Part model, mm, in its own coordinate system. A direction names the side the tool comes from. Give positions to 0.01 mm unless a question says otherwise; leave off trailing zeros. Order: outer loops, then holes, each group sorted by start corner. A loop starts at its lowest first (then second) coordinate and runs counter-clockwise, first axis right, second up. Notation, with made-up numbers: M 25,-24.5 L 53,-24.5 A31 ccw 53,10.5 Z; hole C -3,-2 d2. An arc over 180 degrees is marked long. Answer as a JSON object with one key per item and string values.
from build123d import *

# Parameters (mm, degrees)
SKIZZE1_R                       = 19
SKIZZE1_R_2                     = 1.6
AUFSATZ_LINEAR_AUSTRAGEN1_DEPTH = 3
SKIZZE6_R                       = 3
SCHNITT_LINEAR_AUSTRAGEN2_DEPTH = 36.482389998
SKIZZE7_W                       = 3
SKIZZE7_H                       = 12
SKIZZE7_W_2                     = 12
SKIZZE7_H_2                     = 3
SCHNITT_LINEAR_AUSTRAGEN3_DEPTH = 1.2


with BuildPart() as part:
    # Skizze1 → Aufsatz-Linear austragen1 (new body)
    with BuildSketch(Plane(origin=(0, 0, 0), x_dir=(1, 0, 0), z_dir=(0, 1, 0))):
        with BuildLine():
            ThreePointArc((6, -20.493901532), (6.348554352, -19.365749382), (7.272727273, -18.630819574))
            ThreePointArc((7.272727273, -18.630819574), (14.142135624, -14.142135624), (18.630819574, -7.272727273))
            ThreePointArc((18.630819574, -7.272727273), (19.365749382, -6.348554352), (20.493901532, -6))
            Line((20.493901532, -6), (22.649503306, -6))
            ThreePointArc((22.649503306, -6), (23.93487248, -5.532261755), (24.619025332, -4.347826087))
            ThreePointArc((24.619025332, -4.347826087), (25, 0), (24.619025332, 4.347826087))
            ThreePointArc((24.619025332, 4.347826087), (23.93487248, 5.532261755), (22.649503306, 6))
            Line((22.649503306, 6), (20.493901532, 6))
            ThreePointArc((20.493901532, 6), (19.365749382, 6.348554352), (18.630819574, 7.272727273))
            ThreePointArc((18.630819574, 7.272727273), (14.142135624, 14.142135624), (7.272727273, 18.630819574))
            ThreePointArc((7.272727273, 18.630819574), (6.348554352, 19.365749382), (6, 20.493901532))
            Line((6, 20.493901532), (6, 22.649503306))
            ThreePointArc((6, 22.649503306), (5.532261755, 23.93487248), (4.347826087, 24.619025332))
            ThreePointArc((4.347826087, 24.619025332), (0, 25), (-4.347826087, 24.619025332))
            ThreePointArc((-4.347826087, 24.619025332), (-5.532261755, 23.93487248), (-6, 22.649503306))
            Line((-6, 22.649503306), (-6, 20.493901532))
            ThreePointArc((-6, 20.493901532), (-6.348554352, 19.365749382), (-7.272727273, 18.630819574))
            ThreePointArc((-7.272727273, 18.630819574), (-14.142135624, 14.142135624), (-18.630819574, 7.272727273))
            ThreePointArc((-18.630819574, 7.272727273), (-19.365749382, 6.348554352), (-20.493901532, 6))
            Line((-20.493901532, 6), (-22.649503306, 6))
            ThreePointArc((-22.649503306, 6), (-23.93487248, 5.532261755), (-24.619025332, 4.347826087))
            ThreePointArc((-24.619025332, 4.347826087), (-25, 0), (-24.619025332, -4.347826087))
            ThreePointArc((-24.619025332, -4.347826087), (-23.93487248, -5.532261755), (-22.649503306, -6))
            Line((-22.649503306, -6), (-20.493901532, -6))
            ThreePointArc((-20.493901532, -6), (-19.365749382, -6.348554352), (-18.630819574, -7.272727273))
            ThreePointArc((-18.630819574, -7.272727273), (-14.142135624, -14.142135624), (-7.272727273, -18.630819574))
            ThreePointArc((-7.272727273, -18.630819574), (-6.348554352, -19.365749382), (-6, -20.493901532))
            Line((-6, -20.493901532), (-6, -22.649503306))
            ThreePointArc((-6, -22.649503306), (-5.532261755, -23.93487248), (-4.347826087, -24.619025332))
            ThreePointArc((-4.347826087, -24.619025332), (0, -25), (4.347826087, -24.619025332))
            ThreePointArc((4.347826087, -24.619025332), (5.532261755, -23.93487248), (6, -22.649503306))
            Line((6, -22.649503306), (6, -20.493901532))
        make_face()
        Circle(SKIZZE1_R, mode=Mode.SUBTRACT)
        Circle(SKIZZE1_R)
        with Locations(Location((0, -10, 0), (0, 0, 270))):
            Circle(SKIZZE1_R_2, mode=Mode.SUBTRACT)
        with Locations(Location((-10, 0, 0), (0, 0, 270))):
            Circle(SKIZZE1_R_2, mode=Mode.SUBTRACT)
        with Locations(Location((10, 0, 0), (0, 0, 270))):
            Circle(SKIZZE1_R_2, mode=Mode.SUBTRACT)
        with Locations(Location((0, 10, 0), (0, 0, 270))):
            Circle(SKIZZE1_R_2, mode=Mode.SUBTRACT)
        with Locations(Location((0, 0, 0), (0, 0, 270))):
            Circle(SKIZZE1_R_2, mode=Mode.SUBTRACT)
    extrude(amount=AUFSATZ_LINEAR_AUSTRAGEN1_DEPTH)

    # Skizze6 → Schnitt-Linear austragen2 (cut, through all)
    with BuildSketch(Plane.XZ):
        with Locations(Location((0, 0, 0), (0, 0, 270))):
            Circle(SKIZZE6_R)
    extrude(amount=-SCHNITT_LINEAR_AUSTRAGEN2_DEPTH, mode=Mode.SUBTRACT)

    # Skizze7 → Schnitt-Linear austragen3 (cut)
    with BuildSketch(Plane.XZ):
        with Locations((-22.119025332, 0)):
            Rectangle(SKIZZE7_W, SKIZZE7_H)
        with Locations((0, 22.119025332)):
            Rectangle(SKIZZE7_W_2, SKIZZE7_H_2)
        with Locations((22.119025332, 0)):
            Rectangle(SKIZZE7_W, SKIZZE7_H)
        with Locations((0, -22.119025332)):
            Rectangle(SKIZZE7_W_2, SKIZZE7_H_2)
    extrude(amount=-SCHNITT_LINEAR_AUSTRAGEN3_DEPTH, mode=Mode.SUBTRACT)


solid = part.part
1. Cut at C-C on x = 10. Give the cut face in (y, z), plus the area to 3 significant figures.
Worked answers:
{"outline": "M 0,-17.32 L 3,-17.32 L 3,-1.6 L 0,-1.6 Z; M 0,1.6 L 3,1.6 L 3,17.32 L 0,17.32 Z", "area": "94.3 mm^2"}
2. Probe line 1 along X through (y, z) = (0.75, 5); line 2 along Z through (x, y) = (0.5, 0.9) (3 decimals); line 3 along X through (y, z) = (2.7, -20.5). List the from-to ranges inside material, lowest first.
Worked answers:
{"line 1": "x = -24.38 to -23.62, -20.62 to 20.62, 23.62 to 24.38", "line 2": "z = -24.995 to -23.619, -20.619 to -11.52, -8.48 to -2.958, 2.958 to 8.48, 11.52 to 20.619, 23.619 to 24.995", "line 3": "x = -6 to 6"}
3. Cut at B-B on z = 0. Give the cut face in (x, y), plus the area to 3 significant figures.
Worked answers:
{"outline": "M -25,0 L -23.62,0 L -23.62,1.2 L -20.62,1.2 L -20.62,0 L -11.6,0 L -11.6,3 L -25,3 Z; M -8.4,0 L -3,0 L -3,3 L -8.4,3 Z; M 3,0 L 8.4,0 L 8.4,3 L 3,3 Z; M 11.6,0 L 20.62,0 L 20.62,1.2 L 23.62,1.2 L 23.62,0 L 25,0 L 25,3 L 11.6,3 Z", "area": "106 mm^2"}
4. Pin check, flat tips, straight feed: P1, Ø0.6, axis at y = 0.5, z = 2.5, coming from the +X side; P2, Ø1.1, axis at y = 2, z = -21.5, coming from the -X side; P3, Ø1.7, axis at y = 2, z = 21, coming from the +X side; P4, Ø1.9, axis at x = -10, z = 0, coming from the +Y side. Stop position of each tip, or through.
Worked answers:
{"P1": "stops at x = 24.9", "P2": "stops at x = -6", "P3": "stops at x = 6.03", "P4": "passes through"}
5. Which spindle directions (+Z, -Z, +X, -X, +Y, -Y) get a long thin tool onto all of the face, cutting with end or side? Do faces 5 (the flat face through (22, 1.2, 0)), 6 (the flat face through (-22, 2, -6)), 7 (the flat face through (-22, 2, 6)), 8 (the flat face through (0, 1, 23.619)). Say none if no direction does.
Worked answers:
{"face 5": "+Z, -Z, -Y", "face 6": "-Z, -X, +Y, -Y", "face 7": "+Z, -X, +Y, -Y", "face 8": "+X, -X, -Y"}
6. Cut at A-A on y = 0.6. State how many separate pieces and enclosed holes the cut face has, plus the area to 3 significant figures.
Worked answers:
{"separate pieces": "5", "enclosed holes": "5", "area": "1,290 mm^2"}
7. Two-plate mould, pull along Z, no slides. Class faces 1 (the flat face through (0, 1.2, -22)), 2 (the cylindrical face through (19.35, 1.48, 6.36)), 3 (the cylindrical face through (6.36, 1.48, -19.35)), 4 (the cylindrical face through (0.9, 1.48, -2.86)): +Z half, -Z half, draft (parallel to the pull), parting line (faces both ways), or undercut.
Worked answers:
{"face 1": "undercut", "face 2": "+Z half", "face 3": "-Z half", "face 4": "undercut"}
8. Cut at D-D on x = -1. Give the cut face in (y, z), plus the area to 3 significant figures.
Worked answers:
{"outline": "M 0,-24.98 L 3,-24.98 L 3,-11.25 L 0,-11.25 L 0,-20.62 L 1.2,-20.62 L 1.2,-23.62 L 0,-23.62 Z; M 0,-8.75 L 3,-8.75 L 3,-2.83 L 0,-2.83 Z; M 0,2.83 L 3,2.83 L 3,8.75 L 0,8.75 Z; M 0,11.25 L 3,11.25 L 3,24.98 L 0,24.98 L 0,23.62 L 1.2,23.62 L 1.2,20.62 L 0,20.62 Z", "area": "111 mm^2"}
